For this review, take the finished solid that the model builds, in its own axes (mm). Coordinates: 2 decimals unless noted, no trailing zeros. Order: outer loops, then holes, each group sorted by start corner. A loop starts at its lowest first (then second) coordinate and runs counter-clockwise, first axis right, second up. Notation, with made-up numbers: (52, -20.75) -> (72, -20.75) arc R23 cw to (72, 17.25) -> close; hole circle Ø2 at (-30, 29.25). An arc over 180 degrees is marked (long way). Write item = value, one per line. Start each with the question number.
1) Consider section D-D on x = -86. Give the boundary of the cut face in (y, z).
2) Consider section A-A on x = -55. Give the boundary of the cut face in (y, z).
3) Wall thickness on probe 1 along Y at (x, z) = (55, 2.45); probe 2 along X at (y, z) = (-34, 2.8); probe 3 along X at (y, z) = (-25.5, 1.4): over which ranges is each line inside the solid? List them lowest first. Write a range as [from, to].
4) Consider section C-C on z = 2.5. State how many separate pieces and enclosed holes the cut face has, and give its area (3 significant figures).
5) Insertion check: pin 1 Ø5 at (x, y) = (55, -55) entering from +Z; pin 2 Ø0.9 at (y, z) = (42, 2) entering from -X; pin 3 Ø0.9 at (y, z) = (46.5, 1) entering from +X; pin 4 Ø1.5 at (x, z) = (35.5, 2) entering from +Y. Each pin has a flat end and moves straight along its axis. Give the tip position at first contact, or say it passes through.
6) Consider section B-B on y = -61.5. Give the boundary of the cut face in (x, z), and give its area (3 significant figures).
7) Draft analysis for pull direction Y (two halves, no side actions). For faces 1 (the face through (57.027, 56.859, 1.479)), 2 (the face through (-1, 1, 0)), 3 (the face through (95.38, 30.04, 1.48)), state which applies: +Y half, -Y half, draft (parallel to the pull), parting line (faces both ways), or undercut.
from build123d import *

# Parameters (mm, degrees)
IZIM1_R                     = 100
Y_KSEKLIK_EKSTR_ZYON1_DEPTH = 30
KES_EKSTR_ZYON1_DEPTH       = 145.568322948
M5_BO_LUKLU_DELIK2_D        = 5.5
IZIM20_R                    = 183.537558205
KES_EKSTR_ZYON3_DEPTH       = 27


with BuildPart() as part:
    # Çizim1 → Yükseklik-Ekstrüzyon1 (new body)
    with BuildSketch(Plane.XY):
        Circle(IZIM1_R)
    extrude(amount=Y_KSEKLIK_EKSTR_ZYON1_DEPTH)

    # Çizim9 → Kes-Ekstrüzyon1 (cut, through all)
    with BuildSketch(Plane.XY.offset(30)):
        with BuildLine():
            Line((27, 65), (27, 25))
            ThreePointArc((27, 25), (23.5, 21.5), (20, 25))
            Line((20, 25), (20, 65))
            ThreePointArc((20, 65), (23.5, 68.5), (27, 65))
        make_face()
        with BuildLine():
            Line((-20, 65), (-20, 25))
            ThreePointArc((-20, 25), (-23.5, 21.5), (-27, 25))
            Line((-27, 25), (-27, 65))
            ThreePointArc((-27, 65), (-23.5, 68.5), (-20, 65))
        make_face()
        with BuildLine():
            Line((-20, -25), (-20, -65))
            ThreePointArc((-20, -65), (-23.5, -68.5), (-27, -65))
            Line((-27, -65), (-27, -25))
            ThreePointArc((-27, -25), (-23.5, -21.5), (-20, -25))
        make_face()
        with BuildLine():
            Line((20, -65), (20, -25))
            ThreePointArc((20, -25), (23.5, -21.5), (27, -25))
            Line((27, -25), (27, -65))
            ThreePointArc((27, -65), (23.5, -68.5), (20, -65))
        make_face()
    extrude(amount=-KES_EKSTR_ZYON1_DEPTH, mode=Mode.SUBTRACT)

    # M5 Boşluklu Delik2 (through all)
    with Locations(Plane.XY.offset(30)):
        with Locations((-55, 55), (55, 55), (55, -55), (-55, -55)):
            Hole(M5_BO_LUKLU_DELIK2_D / 2)

    # Çizim20 → Kes-Ekstrüzyon3 (cut)
    with BuildSketch(Plane.XY.offset(30)):
        with Locations((0, 8.479468632)):
            Circle(IZIM20_R)
    extrude(amount=-KES_EKSTR_ZYON3_DEPTH, mode=Mode.SUBTRACT)


solid = part.part
Answer sheet:
q1.outline = (-51.03, 0) -> (51.03, 0) -> (51.03, 3) -> (-51.03, 3) -> close
q2.outline = (-83.52, 0) -> (-57.75, 0) -> (-57.75, 3) -> (-83.52, 3) -> close; (-52.25, 0) -> (52.25, 0) -> (52.25, 3) -> (-52.25, 3) -> close; (57.75, 0) -> (83.52, 0) -> (83.52, 3) -> (57.75, 3) -> close
q3.probe_1 = [-83.52, -57.75], [-52.25, 52.25], [57.75, 83.52]
q3.probe_2 = [-94.04, -27], [-20, 20], [27, 94.04]
q3.probe_3 = [-96.69, -27], [-20, 20], [27, 96.69]
q4.separate_pieces = 1
q4.enclosed_holes = 8
q4.area = 30,000 mm2
q5.pin_1 = through
q5.pin_2 = -90.96
q5.pin_3 = 88.77
q5.pin_4 = 93.77
q6.outline = (-78.85, 0) -> (-27, 0) -> (-27, 3) -> (-78.85, 3) -> close; (-20, 0) -> (20, 0) -> (20, 3) -> (-20, 3) -> close; (27, 0) -> (78.85, 0) -> (78.85, 3) -> (27, 3) -> close
q6.area = 431 mm2
q7.face_1 = undercut
q7.face_2 = draft
q7.face_3 = parting line
